Read the model definition and answer for the solid it produces. Units are mm, in the model's axes. Coordinates: 2 decimals unless noted, no trailing zeros. Loops run counter-clockwise (first coordinate to the right, second up) from the corner with the lowest first, then second, coordinate; pieces in that order, holes last.
from build123d import *

# Parameters (mm, degrees)
F0_R     = 38.1
F1_DEPTH = 6.35
F2_T     = -2.54
F3_R     = 5.08


with BuildPart() as f1:
    # F0 (on Top) → F1 (new body, symmetric)
    with BuildSketch(Plane.XY):
        Circle(F0_R)
    extrude(amount=F1_DEPTH, both=True)

    # F2
    f2_openings = [f1.faces().sort_by_distance(p)[0] for p in [
        (0, 0, 6.35),
    ]]
    offset(amount=F2_T, openings=f2_openings)

    # F3
    f3_edges = [f1.edges().sort_by_distance(p)[0] for p in [
        (-35.56, 0, -3.81),
    ]]
    fillet(f3_edges, radius=F3_R)


solid = f1.part
Item 1: A cutting plane is placed at D-D on z = -2. Determine the outline of the cut face in (x, y), then the cut area to 3 significant figures.
Numbers:
outline: circle Ø76.2 at (0, 0); hole circle Ø68.74 at (0, 0)
area: 850 mm2
Item 2: Find the intervals of material crossed by line 1 along Y through (x, z) = (0, 4.3); line 2 along Z through (x, y) = (-5.5, -4); line 3 along Y through (x, z) = (-2, -0.75), in increasing order.
Numbers:
line 1: y = -38.1 to -35.56, 35.56 to 38.1
line 2: z = -6.35 to -3.81
line 3: y = -38.05 to -35.08, 35.08 to 38.05
Item 3: A cutting plane is placed at C-C on z = 5. Determine the outline of the cut face in (x, y), then the cut area to 3 significant figures.
Numbers:
outline: circle Ø76.2 at (0, 0); hole circle Ø71.12 at (0, 0)
area: 588 mm2
Item 4: Determine the mould class of faces 1 (the face through (-1, 1, -6.35)), 2 (the face through (-30.235, -23.183, 0.089)), 3 (the face through (-7.709, -34.714, 3.846)), 4 (the face through (0, 0, -3.81)) for opening direction X: released by +X, released by -X, zero draft, split by the parting line, or undercut.
Numbers:
face 1: zero draft
face 2: split by the parting line
face 3: undercut
face 4: undercut
Item 5: A cutting plane is placed at A-A on x = 0. Determine the outline of the cut face in (y, z).
Numbers:
outline: (-38.1, -6.35) - (38.1, -6.35) - (38.1, 6.35) - (35.56, 6.35) - (35.56, 1.27) arc R5.08 cw to (30.48, -3.81) - (-30.48, -3.81) arc R5.08 cw to (-35.56, 1.27) - (-35.56, 6.35) - (-38.1, 6.35) - close
Item 6: Given pin 1 (2 mm diameter, centred on x = -26.5, z = 3, fed in from -Y); pin 2 (3 mm diameter, centred on y = -12.5, z = -0.5, fed in from +X); pin 3 (2 mm diameter, centred on y = 11, z = -2, fed in from -X), each flat-ended and moving along its own axis, determine where each tip first touches the part or whether it passes through.
Numbers:
pin 1: stops at y = -28.31
pin 2: stops at x = 36.48
pin 3: stops at x = -36.76
